from build123d import *

# Parameters (mm, degrees)
ESBO_O2_R                = 3
RESSALTO_EXTRUS_O1_DEPTH = 20
ESBO_O3_R                = 6
CORTE_EXTRUS_O1_DEPTH    = 17


with BuildPart() as part:
    # Esboço2 → Ressalto-extrusão1 (new body)
    with BuildSketch(Plane.XY):
        Polygon((-8.660254038, 5), (-8.660254038, -5), (0, -10), (8.660254038, -5), (8.660254038, 5), (0, 10), align=None)
        Circle(ESBO_O2_R, mode=Mode.SUBTRACT)
    extrude(amount=RESSALTO_EXTRUS_O1_DEPTH)

    # Esboço3 → Corte-extrusão1 (cut)
    with BuildSketch(Plane(origin=(0, 0, 0), x_dir=(-1, 0, 0), z_dir=(0, 0, -1))):
        Circle(ESBO_O3_R)
    extrude(amount=-CORTE_EXTRUS_O1_DEPTH, mode=Mode.SUBTRACT)

    # Esboço6 → Corte-Revolução3 (revolve, cut)
    with BuildSketch(Plane(origin=(0, 0, 0), x_dir=(1, 0, 0), z_dir=(0, 1, 0))):
        Polygon((-8.660254038, -3.5), (-10.094489548, -3.5), (-10.094489548, -4.5), (-8.660254038, -4.5), (-7.660254038, -4.5), (-7.660254038, -3.5), align=None)
    revolve(axis=Axis((0, 0, 21), (0, 0, -1)), mode=Mode.SUBTRACT)

    # Esboço11 → Corte-Revolução7 (revolve, cut)
    with BuildSketch(Plane(origin=(0, 0, 0), x_dir=(0, 0, -1), z_dir=(1, 0, 0))):
        Polygon((0, 9), (-0.5, 10), (-3, 10), (-3.5, 9), (-4.5, 9), (-5, 10), (-19.5, 10), (-20, 9), (-20, 10.45616239), (0, 10.45616239), align=None)
    revolve(axis=Axis((0, 0, 21), (0, 0, -1)), mode=Mode.SUBTRACT)


solid = part.part
CAD build for the part. Positions are in the model's coordinates, mm. A direction names the side the tool comes from. Round coordinates to 2 decimals unless told otherwise and drop trailing zeros. Write each loop counter-clockwise with the first axis right and the second up, starting at its lowest first coordinate (ties: lowest second). Pieces come first, ordered by that corner, then holes. Notation, with made-up numbers: M -19.75,-30 L -10.75,-30 A26 cw -10.75,-10 Z; hole C 32.5,17 d3. An arc over 180 degrees is marked long. Use a Markdown table: item, result. Add a question column.
1. Slice it at A-A on z = 16.5. Give the cut face in (x, y), then the cut area to 3 significant figures.
2. Pull direction Z, two halves, no side cores. Call faces 1 (the face through (8.057, -4.614, 4.642)), 2 (the face through (-0.03, 9.28, 0.14)), 3 (the face through (0.032, -9.271, 19.865)), 4 (the face through (-0.032, 9.271, 3.365)): released by +Z, released by -Z, zero draft, split by the parting line, or undercut.
3. Flat gauge pins, fed straight in: P1, Ø3, axis at x = -4.5, z = 13, coming from the -Y side; P2, Ø2, axis at x = -5.5, z = 13, coming from the -Y side; P3, Ø3.5, axis at x = 2.5, y = -3, coming from the -Z side. Where does each tip first touch, or does it go through?
4. Drill centre lines: probe 1 along Z at (x, y) = (2, 7.5); probe 2 along X at (y, z) = (0, 19.2); probe 3 along Y at (x, z) = (-1.5, 8.5). Where is each one in solid material? Low to high.
5. Slice it at B-B on y = 0. Give the cut face in (x, z).
6. 3-axis set-ups, long thin cutter, end or side, ignore diameter. For faces 5 (the face through (8.013, 4.663, 3.365)), 6 (the face through (-8.013, -4.663, 3.365)), 7 (the face through (1.66, -7.48, 3.99)), 8 (the face through (-8.057, 4.614, 4.642)): which of +Z, -Z, +X, -X, +Y, -Y reach the whole face in a straight line?
Reply:
| question | item | result |
|---|---|---|
| 1 | outline | M -8.66,-5 L 0,-10 L 8.66,-5 L 8.66,5 L 0,10 L -8.66,5 Z; hole C 0,0 d12 |
| 1 | area | 147 mm^2 |
| 2 | face 1 | undercut |
| 2 | face 2 | released by -Z |
| 2 | face 3 | released by +Z |
| 2 | face 4 | undercut |
| 3 | P1 | stops at y = -8.27 |
| 3 | P2 | stops at y = -7.4 |
| 3 | P3 | stops at z = 17 |
| 4 | probe 1 | z = 0 to 3.5, 4.5 to 20 |
| 4 | probe 2 | x = -8.66 to -3, 3 to 8.66 |
| 4 | probe 3 | y = -9.13 to -5.81, 5.81 to 9.13 |
| 5 | outline | M -8.66,0 L -6,0 L -6,17 L -3,17 L -3,20 L -8.66,20 L -8.66,4.5 L -7.66,4.5 L -7.66,3.5 L -8.66,3.5 Z; M 3,17 L 6,17 L 6,0 L 8.66,0 L 8.66,3.5 L 7.66,3.5 L 7.66,4.5 L 8.66,4.5 L 8.66,20 L 3,20 Z |
| 6 | face 5 | +X, +Y |
| 6 | face 6 | -X, -Y |
| 6 | face 7 | none |
| 6 | face 8 | -X, +Y |
